Autodesk Fusion 360 part; units mm, degrees
sketch "Sketch1" plane through (0, 0, 0) normal (0, 0, 1) x (1, 0, 0)
  line L0 (7, 4.5) -> (7, 0.5)
  line L1 (6.5, 0) -> (0.5, 0)
  arc A0 (6.5, 0) -> (7, 0.5) centre (6.5, 0.5) ccw
  line L2 (0.5, 5.6) -> (6.5, 5.6)
  line L3 (7, 5.1) -> (7, 4.5)
  arc A1 (7, 5.1) -> (6.5, 5.6) centre (6.5, 5.1) ccw
  line L4 (-1, 0.5) -> (-1, 5)
  line L5 (-1, 5) -> (-1, 5.1)
  line L6 (-0.5, 5.6) -> (0.5, 5.6)
  line L7 (-0.5, 0) -> (0.5, 0)
  arc A2 (-0.5, 5.6) -> (-1, 5.1) centre (-0.5, 5.1) ccw
  arc A3 (-1, 0.5) -> (-0.5, 0) centre (-0.5, 0.5) ccw
extrude "Extrude1" add sketch "Sketch1" along normal blind 0.6
sketch "Sketch7" plane through (0, 0, 0.6) normal (0, 0, 1) x (-1, 0, 0)
  line L0 (0.5, 0) -> (-6.5, 0)
  arc A0 (-6.5, 0) -> (-7, -0.5) centre (-6.5, -0.5) ccw
  line L1 (-7, -0.5) -> (-7, -4.5)
  line L2 (-7, -4.5) -> (-7, -5.1)
  arc A1 (-7, -5.1) -> (-6.5, -5.6) centre (-6.5, -5.1) ccw
  line L3 (-6.5, -5.6) -> (0.5, -5.6)
  line L4 (-2.6, -2.8) -> (-2.6, -4.5)
  line L5 (-2.6, -4.5) -> (-6, -4.5)
  line L6 (-6, -4.5) -> (-6, -1.1)
  line L7 (-6, -1.1) -> (-2.6, -1.1)
  line L8 (-2.6, -1.1) -> (-2.6, -2.8)
  line L9 (1, -5.1) -> (1, -0.5)
  arc A2 (1, -0.5) -> (0.5, 0) centre (0.5, -0.5) ccw
  arc A3 (0.5, -5.6) -> (1, -5.1) centre (0.5, -5.1) ccw
  dimension "d30" = 1.7
  dimension "d31" = 3.4
  dimension "d32" = 3.4
extrude "Extrude7" add sketch "Sketch7" along normal blind 2 contours L4 L5 L6 L7 L8
sketch "Sketch8" plane through (0, 0, 2.6) normal (0, 0, 1) x (-1, 0, 0)
  line L0 (-2.6, -1.1) -> (-6, -1.1)
  line L1 (-6, -1.1) -> (-6, -4.5)
  line L2 (-6, -4.5) -> (-2.6, -4.5)
  line L3 (-2.6, -4.5) -> (-2.6, -2.8)
  line L4 (-2.6, -2.8) -> (-2.6, -1.1)
  circle A0 centre (-4.3, -2.8) radius 1
extrude "Extrude8" cut sketch "Sketch8" against normal blind 1 contours A0
sketch "Sketch9" plane through (0, 0, 0.6) normal (0, 0, 1) x (-1, 0, 0)
  line L0 (-2.6, -1.1) -> (-2.6, -2.8)
  line L1 (-2.6, -2.8) -> (-2.6, -4.5)
  line L2 (-2.6, -4.5) -> (-6, -4.5)
  line L3 (-6, -4.5) -> (-6, -1.1)
  line L4 (-6, -1.1) -> (-2.6, -1.1)
  line L5 (-7, -4.5) -> (-7, -5.1)
  arc A0 (-7, -5.1) -> (-6.5, -5.6) centre (-6.5, -5.1) ccw
  line L6 (-6.5, -5.6) -> (0.5, -5.6)
  line L7 (0.5, 0) -> (-6.5, 0)
  arc A1 (-6.5, 0) -> (-7, -0.5) centre (-6.5, -0.5) ccw
  line L8 (-7, -0.5) -> (-7, -4.5)
  line L9 (-1.5, -1.1) -> (0.1, -1.1)
  line L10 (0.1, -1.1) -> (0.1, -1.9)
  line L11 (0.1, -1.9) -> (-1.5, -1.9)
  line L12 (-1.5, -1.9) -> (-1.5, -1.1)
  line L13 (-1.5, -2.6) -> (0.1, -2.6)
  line L14 (0.1, -2.6) -> (0.1, -3.4)
  line L15 (0.1, -3.4) -> (-1.5, -3.4)
  line L16 (-1.5, -3.4) -> (-1.5, -2.6)
  line L17 (1, -5.1) -> (1, -0.5)
  arc A2 (1, -0.5) -> (0.5, 0) centre (0.5, -0.5) ccw
  arc A3 (0.5, -5.6) -> (1, -5.1) centre (0.5, -5.1) ccw
extrude "Extrude9" add sketch "Sketch9" along normal blind 0.8 contours L9 L10 L11 L12 | L13 L14 L15 L16
sketch "Sketch10" plane through (0, 0, 0.6) normal (0, 0, 1) x (-1, 0, 0)
  line L0 (-2.6, -1.1) -> (-2.6, -2.8)
  line L1 (-2.6, -2.8) -> (-2.6, -4.5)
  line L2 (-2.6, -4.5) -> (-6, -4.5)
  line L3 (-6, -4.5) -> (-6, -1.1)
  line L4 (-6, -1.1) -> (-2.6, -1.1)
  line L5 (-7, -4.5) -> (-7, -5.1)
  arc A0 (-7, -5.1) -> (-6.5, -5.6) centre (-6.5, -5.1) ccw
  line L6 (-6.5, -5.6) -> (0.5, -5.6)
  line L7 (0.5, 0) -> (-6.5, 0)
  arc A1 (-6.5, 0) -> (-7, -0.5) centre (-6.5, -0.5) ccw
  line L8 (-7, -0.5) -> (-7, -4.5)
  circle A2 centre (0.2, -4.8) radius 0.3
  circle A3 centre (-1.6, -4.8) radius 0.3
  circle A4 centre (-0.7, -4.1) radius 0.3
  line L9 (-1.5, -1.1) -> (0.1, -1.1)
  line L10 (0.1, -3.4) -> (-1.5, -3.4)
  line L11 (-1.5, -3.4) -> (-1.5, -2.6)
  line L12 (-1.5, -2.6) -> (0.1, -2.6)
  line L13 (0.1, -1.9) -> (-1.5, -1.9)
  line L14 (-1.5, -1.9) -> (-1.5, -1.1)
  line L15 (0.1, -1.1) -> (0.1, -1.9)
  line L16 (0.1, -2.6) -> (0.1, -3.4)
  line L17 (1, -5.1) -> (1, -0.5)
  arc A5 (1, -0.5) -> (0.5, 0) centre (0.5, -0.5) ccw
  arc A6 (0.5, -5.6) -> (1, -5.1) centre (0.5, -5.1) ccw
extrude "Extrude10" cut sketch "Sketch10" against normal blind 0.6 contours A2 | A3 | A4
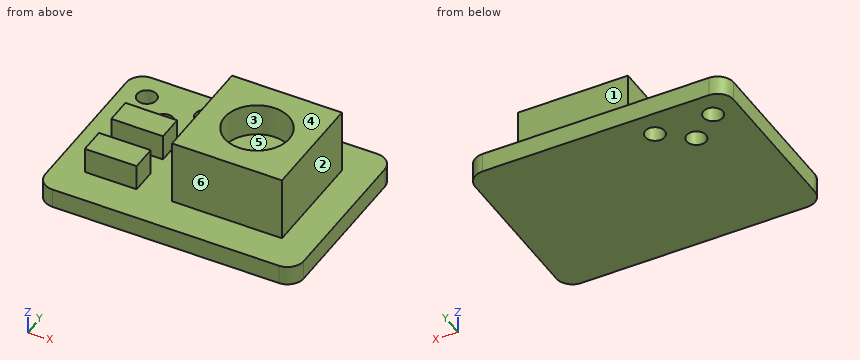
CAD build for the part. Positions are in the model's coordinates, mm. Face numbers are marked on the shaded views. A direction names the side the tool comes from. Coordinates: 2 decimals unless noted, no trailing zeros. Write each loop counter-clockwise with the first axis right and the second up, starting at its lowest first coordinate (ties: lowest second). Pieces come first, ordered by that corner, then holes.
(1) Cut at B-B, the plane x = 0.7. List the corners of the cut face in (y, z), and give its area (3 significant figures).
(2) Cut at C-C, the plane z = 1.1. List the corners of the cut face in (x, y), and give its area (3 significant figures).
(3) 3-axis set-ups, long thin cutter, end or side, ignore diameter. For the marked faces 4, 5 and 6: which of +Z, -Z, +X, -X, +Y, -Y reach the whole face in a straight line?
(4) Cut at D-D, the plane y = 4.8. List the corners of the cut face in (x, z), and give its area (3 significant figures).
(5) Two-plate mould, pull along Y, no slides. Class the marked faces 1, 2 and 3: +Y half, -Y half, draft (parallel to the pull), parting line (faces both ways), or undercut.
(6) Drill centre lines: probe 1 along X at (y, z) = (4.8, 0.25); probe 2 along Y at (x, z) = (0.7, 0.2); probe 3 along X at (y, z) = (3.2, 1.35). Where is each one in solid material? Low to high.
(7) Cut at A-A, the plane y = 4.1. List the corners of the cut face in (x, z).
(8) Flat gauge pins, fed straight in: pin 1 (0.6 mm diameter, centred on x = 3.5, z = 1.5, fed in from +Y); pin 2 (0.6 mm diameter, centred on x = 4.5, z = 1, fed in from -Y); pin 3 (0.6 mm diameter, centred on y = 3, z = 1, fed in from +X). Where does each tip first touch, or does it go through?
Geometry says:
1. outline: (0, 0) - (3.8, 0) - (3.8, 0.6) - (3.4, 0.6) - (3.4, 1.4) - (2.6, 1.4) - (2.6, 0.6) - (1.9, 0.6) - (1.9, 1.4) - (1.1, 1.4) - (1.1, 0.6) - (0, 0.6) - close; (4.4, 0) - (5.6, 0) - (5.6, 0.6) - (4.4, 0.6) - close
1. area: 4.28 mm2
2. outline: (-0.1, 1.1) - (1.5, 1.1) - (1.5, 1.9) - (-0.1, 1.9) - close; (-0.1, 2.6) - (1.5, 2.6) - (1.5, 3.4) - (-0.1, 3.4) - close; (2.6, 1.1) - (6, 1.1) - (6, 4.5) - (2.6, 4.5) - close
2. area: 14.1 mm2
3. face 4: +Z, +X, -X, +Y, -Y
3. face 5: +Z
3. face 6: +Z, +X, -X, -Y
4. outline: (-1, 0) - (-0.5, 0) - (-0.5, 0.6) - (-1, 0.6) - close; (0.1, 0) - (1.3, 0) - (1.3, 0.6) - (0.1, 0.6) - close; (1.9, 0) - (7, 0) - (7, 0.6) - (1.9, 0.6) - close
4. area: 4.08 mm2
5. face 1: +Y half
5. face 2: draft
5. face 3: undercut
6. probe 1: x = -1 to -0.5, 0.1 to 1.3, 1.9 to 7
6. probe 2: y = 0 to 3.8, 4.4 to 5.6
6. probe 3: x = -0.1 to 1.5, 2.6 to 6
7. outline: (-1, 0) - (0.4, 0) - (0.4, 0.6) - (-1, 0.6) - close; (1, 0) - (7, 0) - (7, 0.6) - (6, 0.6) - (6, 2.6) - (2.6, 2.6) - (2.6, 0.6) - (1, 0.6) - close
8. pin 1: stops at y = 4.5
8. pin 2: stops at y = 1.1
8. pin 3: stops at x = 6
